Read the model definition and answer for the solid it produces. Units are mm, in the model's axes. A direction names the side the tool comes from. Round coordinates to 2 decimals unless told otherwise and drop trailing zeros. Loops run counter-clockwise (first coordinate to the right, second up) from the corner with the lowest first, then second, coordinate; pieces in that order, holes last. Notation, with made-up numbers: (-36, 47) -> (-6, 47) arc R21 ccw to (-6, 60) -> close; hole circle Ø10 at (26, -35). An arc over 180 degrees is marked (long way). Put each result on its own line as item: value.
Autodesk Fusion 360 part; units mm, degrees
sketch "Sketch1" plane through (0, 0, 0) normal (0, 0, 1) x (1, 0, 0)
  line L0 (0, 0) -> (23.3, 0)
  line L1 (23.3, 0) -> (23.3, 12.5)
  line L2 (23.3, 12.5) -> (0, 12.5)
  line L3 (0, 12.5) -> (0, 0)
  line L4 (0, 6.25) -> (-2.35, 6.25) construction
  line L5 (23.3, 6.25) -> (25.65, 6.25) construction
  circle A0 centre (-2.35, 6.25) radius 1.45
  circle A1 centre (25.65, 6.25) radius 1.45
  line L6 (-4.8, -2) -> (28.1, -2)
  line L7 (28.1, -2) -> (28.1, 12.5)
  line L8 (28.1, 12.5) -> (-4.8, 12.5)
  line L9 (-4.8, 12.5) -> (-4.8, -2)
  dimension "d1" = 23.3
  dimension "d2" = 12.5
  dimension "d3" = 2.35
  dimension "d4" = 2.35
  dimension "d5" = 2.9
  dimension "d6" = 2.9
  dimension "d7" = 2
  dimension "d8" = 2.45
  dimension "d9" = 2.45
extrude "Extrude1" add sketch "Sketch1" along normal blind 2 contours L0 L1 L3 L6 L7 L8 L9
sketch "Sketch2" plane through (0, 0, 2) normal (0, 0, 1) x (-1, 0, 0)
  circle A0 centre (2.35, -6.25) radius 1.45
  circle A1 centre (-25.65, -6.25) radius 1.45
  line L0 (0, -12.5) -> (4.8, -12.5)
  line L1 (4.8, -12.5) -> (4.8, 2)
  line L2 (4.8, 2) -> (-28.1, 2)
  line L3 (-28.1, 2) -> (-28.1, -12.5)
  line L4 (-28.1, -12.5) -> (-23.3, -12.5)
  line L5 (-23.3, -12.5) -> (-23.3, 0)
  line L6 (-23.3, 0) -> (0, 0)
  line L7 (0, 0) -> (0, -12.5)
Item 1: The part is cut by section C-C (y = 6.25). Determine the outline of the cut face in (x, z), then the cut area to 3 significant figures.
Derived:
outline: (-4.8, 0) -> (-3.8, 0) -> (-3.8, 2) -> (-4.8, 2) -> close; (-0.9, 0) -> (0, 0) -> (0, 2) -> (-0.9, 2) -> close; (23.3, 0) -> (24.2, 0) -> (24.2, 2) -> (23.3, 2) -> close; (27.1, 0) -> (28.1, 0) -> (28.1, 2) -> (27.1, 2) -> close
area: 7.60 mm^2
Item 2: The part is cut by section A-A (x = -2.35). Determine the outline of the cut face in (y, z), then the cut area to 3 significant figures.
Derived:
outline: (-2, 0) -> (4.8, 0) -> (4.8, 2) -> (-2, 2) -> close; (7.7, 0) -> (12.5, 0) -> (12.5, 2) -> (7.7, 2) -> close
area: 23.2 mm^2
Item 3: For a pull along Y with two mould halves and no side action, classify faces 3 (the flat face through (-2, 12.5, 1)), 4 (the flat face through (13, -1, 0)), 5 (the cylindrical face through (27.03, 5.81, 0.99)) as pulls with the +Y half, pulls with the -Y half, needs draft (parallel to the pull), parting line crosses it, or undercut.
Derived:
face 3: pulls with the +Y half
face 4: needs draft
face 5: undercut
Item 4: Find the intervals of material crossed by line 1 along X through (y, z) = (11.5, 1.4); line 2 along Y through (x, z) = (-2.35, 0.55); line 3 along X through (y, z) = (5.75, 0.3), in increasing order.
Derived:
line 1: x = -4.8 to 0, 23.3 to 28.1
line 2: y = -2 to 4.8, 7.7 to 12.5
line 3: x = -4.8 to -3.71, -0.99 to 0, 23.3 to 24.29, 27.01 to 28.1
Item 5: The part is cut by section D-D (z = 1.5). Determine the outline of the cut face in (x, y), then the cut area to 3 significant figures.
Derived:
outline: (-4.8, -2) -> (28.1, -2) -> (28.1, 12.5) -> (23.3, 12.5) -> (23.3, 0) -> (0, 0) -> (0, 12.5) -> (-4.8, 12.5) -> close; hole circle Ø2.9 at (-2.35, 6.25); hole circle Ø2.9 at (25.65, 6.25)
area: 173 mm^2
Item 6: The part is cut by section B-B (y = 3). Determine the outline of the cut face in (x, z).
Derived:
outline: (-4.8, 0) -> (0, 0) -> (0, 2) -> (-4.8, 2) -> close; (23.3, 0) -> (28.1, 0) -> (28.1, 2) -> (23.3, 2) -> close
Item 7: Which of the six approach directions +Z, -Z, +X, -X, +Y, -Y give full straight-line access (tool end or side, diameter ignored) to faces 1 (the flat face through (13, -1, 2)), 2 (the flat face through (0, 6, 1))?
Derived:
face 1: +Z, +X, -X, +Y, -Y
face 2: +Z, -Z, +Y
